Part model, mm, in its own coordinate system. Face numbers are marked on the shaded views. A direction names the side the tool comes from. Round coordinates to 2 decimals unless told otherwise and drop trailing zeros. Write each loop counter-clockwise with the first axis right and the second up, starting at its lowest first coordinate (ties: lowest second). Pieces come first, ordered by that corner, then holes.
```python
from build123d import *

# Parameters (mm, degrees)
BOSS_EXTRUDE1_DEPTH    = 8
SPLIT1_SURFACE_1_BACK  = 343.199
SPLIT1_SURFACE_1_DEPTH = 686.398
SPLIT1_SURFACE_2_BACK  = 343.199
SPLIT1_SURFACE_2_DEPTH = 686.398
SKETCH5_R              = 2.5
CUT_EXTRUDE6_DEPTH     = 5.2
SKETCH4_R              = 2.5
CUT_EXTRUDE7_DEPTH     = 10
SKETCH6_R              = 1.5
CUT_EXTRUDE8_DEPTH     = 342.206659287
SKETCH7_W              = 49
SKETCH7_H              = 49
SKETCH7_W_2            = 18
SKETCH7_H_2            = 18
BOSS_EXTRUDE2_DEPTH    = 15
SKETCH8_W              = 49
SKETCH8_H              = 49
SKETCH8_R              = 1.5
BOSS_EXTRUDE3_DEPTH    = 10
SKETCH9_W              = 49
SKETCH9_H              = 49
CUT_EXTRUDE9_DEPTH     = 8
SKETCH10_W             = 49
SKETCH10_H             = 49
SKETCH10_W_2           = 18
SKETCH10_H_2           = 18
BOSS_EXTRUDE4_DEPTH    = 8
SKETCH12_R             = 2.5
CUT_EXTRUDE10_DEPTH    = 343.027753759


with BuildPart() as part:
    # Sketch1 → Boss-Extrude1 (new body)
    with BuildSketch(Plane.XY):
        with BuildLine():
            Line((70, 309.985818768), (85.299227191, 309.985818768))
            ThreePointArc((85.299227191, 309.985818768), (88.489017574, 308.836174247), (90.211957942, 305.915913694))
            Line((90.211957942, 305.915913694), (96.672728921, 271.790334282))
            ThreePointArc((96.672728921, 271.790334282), (97.06575438, 270.906904614), (97.621470019, 270.115641625))
            Line((97.621470019, 270.115641625), (139.950460317, 220.786053348))
            ThreePointArc((139.950460317, 220.786053348), (141.739336996, 217.746026552), (142.361429131, 214.274017901))
            Line((142.361429131, 214.274017901), (142.361429131, 30.859943174))
            ThreePointArc((142.361429131, 30.859943174), (140.896963037, 27.324409268), (137.361429131, 25.859943174))
            Line((137.361429131, 25.859943174), (114.717190871, 25.782318449))
            ThreePointArc((114.717190871, 25.782318449), (112.681998989, 25.341726514), (111.002773989, 24.110332733))
            Line((111.002773989, 24.110332733), (89.38285929, 0))
            Line((89.38285929, 0), (50.5, 0))
            Line((50.5, 0), (28.997226011, 24.110332733))
            ThreePointArc((28.997226011, 24.110332733), (27.318001011, 25.341726514), (25.282809129, 25.782318449))
            Line((25.282809129, 25.782318449), (2.638570869, 25.859943174))
            ThreePointArc((2.638570869, 25.859943174), (-0.896963037, 27.324409268), (-2.361429131, 30.859943174))
            Line((-2.361429131, 30.859943174), (-2.361429131, 214.274017901))
            ThreePointArc((-2.361429131, 214.274017901), (-1.739336996, 217.746026552), (0.049539683, 220.786053348))
            Line((0.049539683, 220.786053348), (42.261389271, 270.115641625))
            ThreePointArc((42.261389271, 270.115641625), (42.81710491, 270.906904614), (43.210130369, 271.790334282))
            Line((43.210130369, 271.790334282), (49.724618218, 305.923183314))
            ThreePointArc((49.724618218, 305.923183314), (51.449026762, 308.838533573), (54.635967087, 309.985818768))
            Line((54.635967087, 309.985818768), (70, 309.985818768))
        make_face()
        with BuildLine():
            Line((15.218798766, 54.807228462), (17.702103505, 54.807228462))
            ThreePointArc((17.702103505, 54.807228462), (21.420312934, 56.347361236), (22.960445707, 60.065570665))
            Line((22.960445707, 60.065570665), (22.960445707, 189.807228462))
            ThreePointArc((22.960445707, 189.807228462), (21.495979613, 193.342762368), (17.960445707, 194.807228462))
            Line((17.960445707, 194.807228462), (14.960456564, 194.807228462))
            ThreePointArc((14.960456564, 194.807228462), (11.424922658, 193.342762368), (9.960456564, 189.807228462))
            Line((9.960456564, 189.807228462), (9.960456564, 60.065570665))
            ThreePointArc((9.960456564, 60.065570665), (11.500589337, 56.347361236), (15.218798766, 54.807228462))
        make_face(mode=Mode.SUBTRACT)
        with BuildLine():
            Line((125.039543436, 54.807228462), (122.039554293, 54.807228462))
            ThreePointArc((122.039554293, 54.807228462), (118.504020387, 56.271694556), (117.039554293, 59.807228462))
            Line((117.039554293, 59.807228462), (117.039554293, 189.807228462))
            ThreePointArc((117.039554293, 189.807228462), (118.504020387, 193.342762368), (122.039554293, 194.807228462))
            Line((122.039554293, 194.807228462), (125.039543436, 194.807228462))
            ThreePointArc((125.039543436, 194.807228462), (128.575077342, 193.342762368), (130.039543436, 189.807228462))
            Line((130.039543436, 189.807228462), (130.039543436, 59.807228462))
            ThreePointArc((130.039543436, 59.807228462), (128.575077342, 56.271694556), (125.039543436, 54.807228462))
        make_face(mode=Mode.SUBTRACT)
    extrude(amount=BOSS_EXTRUDE1_DEPTH)


with BuildPart() as body_2:
    # Split1: the piece behind the surface
    add(part.part)
    # Split1 surface: a surface, the sketch's curves swept straight by 686.398 mm
    with BuildLine(Plane(origin=(0, 0, 0), x_dir=(-1, 0, 0), z_dir=(0, 0, -1)).offset(-SPLIT1_SURFACE_1_BACK), mode=Mode.PRIVATE) as split1_surface_1_path:
        Line((-142.361429131, 144.05225917), (2.361429131, 144.05225917))
    split1_surface_1 = Shell.extrude(split1_surface_1_path.wire(), (0 * SPLIT1_SURFACE_1_DEPTH, 0 * SPLIT1_SURFACE_1_DEPTH, -1 * SPLIT1_SURFACE_1_DEPTH))
    split(bisect_by=split1_surface_1, keep=Keep.BOTTOM)

    # Sketch5 → Cut-Extrude6 (cut)
    with BuildSketch(Plane(origin=(0, 144.05225917, -115.359943174), x_dir=(1, 0, 0), z_dir=(0, -1, 0))):
        with Locations(Location((70, 119.359943174, 0), (0, 0, 270))):
            Circle(SKETCH5_R)
        with Locations(Location((40, 119.359943174, 0), (0, 0, 270))):
            Circle(SKETCH5_R)
        with Locations(Location((2.638570869, 119.359943174, 0), (0, 0, 270))):
            Circle(SKETCH5_R)
    extrude(amount=CUT_EXTRUDE6_DEPTH, mode=Mode.SUBTRACT)


with BuildPart() as part_1:
    add(part.part)

    # Split1: split by a surface, the side it looks to stays
    # Split1 surface: a surface, the sketch's curves swept straight by 686.398 mm
    with BuildLine(Plane(origin=(0, 0, 0), x_dir=(-1, 0, 0), z_dir=(0, 0, -1)).offset(-SPLIT1_SURFACE_2_BACK), mode=Mode.PRIVATE) as split1_surface_2_path:
        Line((-142.361429131, 144.05225917), (2.361429131, 144.05225917))
    split1_surface_2 = Shell.extrude(split1_surface_2_path.wire(), (0 * SPLIT1_SURFACE_2_DEPTH, 0 * SPLIT1_SURFACE_2_DEPTH, -1 * SPLIT1_SURFACE_2_DEPTH))
    split(bisect_by=split1_surface_2, keep=Keep.TOP)

    # Sketch4 → Cut-Extrude7 (cut)
    with BuildSketch(Plane(origin=(0, 144.05225917, 0), x_dir=(-1, 0, 0), z_dir=(0, -1, 0))):
        with Locations(Location((-70, -4, 0), (0, 0, 270))):
            Circle(SKETCH4_R)
        with Locations(Location((-40, -4, 0), (0, 0, 270))):
            Circle(SKETCH4_R)
        with Locations(Location((-100, -4, 0), (0, 0, 270))):
            Circle(SKETCH4_R)
        with Locations(Location((-137.361429131, -4, 0), (0, 0, 90))):
            Circle(SKETCH4_R)
        with Locations(Location((-3.799513716, -4, 0), (0, 0, 270))):
            Circle(SKETCH4_R)
    extrude(amount=-CUT_EXTRUDE7_DEPTH, mode=Mode.SUBTRACT)

    # Sketch6 → Cut-Extrude8 (cut, through all)
    with BuildSketch(Plane.XY.offset(8)):
        with Locations((50.000130369, 267.980334282)):
            Circle(SKETCH6_R)
        with Locations((90.000130369, 267.980334282)):
            Circle(SKETCH6_R)
        with Locations((90.000130369, 227.980334282)):
            Circle(SKETCH6_R)
        with Locations((50.000130369, 227.980334282)):
            Circle(SKETCH6_R)
    extrude(amount=-CUT_EXTRUDE8_DEPTH, mode=Mode.SUBTRACT)

    # Sketch7 → Boss-Extrude2 (add)
    with BuildSketch(Plane(origin=(0, 0, 0), x_dir=(-1, 0, 0), z_dir=(0, 0, -1))):
        with Locations((-70.000130369, 247.980334282)):
            Rectangle(SKETCH7_W, SKETCH7_H)
        with Locations((-56.000130369, 261.980334282)):
            Rectangle(SKETCH7_W_2, SKETCH7_H_2, mode=Mode.SUBTRACT)
        with Locations((-84.000130369, 261.980334282)):
            Rectangle(SKETCH7_W_2, SKETCH7_H_2, mode=Mode.SUBTRACT)
        with Locations((-84.000130369, 233.980334282)):
            Rectangle(SKETCH7_W_2, SKETCH7_H_2, mode=Mode.SUBTRACT)
        with Locations((-56.000130369, 233.980334282)):
            Rectangle(SKETCH7_W_2, SKETCH7_H_2, mode=Mode.SUBTRACT)
    extrude(amount=BOSS_EXTRUDE2_DEPTH)

    # Sketch8 → Boss-Extrude3 (add)
    with BuildSketch(Plane(origin=(0, 0, -15), x_dir=(-1, 0, 0), z_dir=(0, 0, -1))):
        with Locations((-70.000130369, 247.980334282)):
            Rectangle(SKETCH8_W, SKETCH8_H)
        with Locations(Location((-50.000130369, 267.980334282, 0), (0, 0, 180))):
            Circle(SKETCH8_R, mode=Mode.SUBTRACT)
        with Locations(Location((-90.000130369, 267.980334282, 0), (0, 0, 180))):
            Circle(SKETCH8_R, mode=Mode.SUBTRACT)
        with Locations(Location((-50.000130369, 227.980334282, 0), (0, 0, 180))):
            Circle(SKETCH8_R, mode=Mode.SUBTRACT)
        with Locations(Location((-90.000130369, 227.980334282, 0), (0, 0, 180))):
            Circle(SKETCH8_R, mode=Mode.SUBTRACT)
    extrude(amount=BOSS_EXTRUDE3_DEPTH)

    # Sketch9 → Cut-Extrude9 (cut)
    with BuildSketch(Plane.XY.offset(8)):
        with Locations((70.000130369, 247.980334282)):
            Rectangle(SKETCH9_W, SKETCH9_H)
    extrude(amount=-CUT_EXTRUDE9_DEPTH, mode=Mode.SUBTRACT)


with BuildPart() as cut_extrude9_piece_1:
    # of the separate pieces the step leaves, piece 1, a body of its own (cut_extrude9_pieces)
    add(part_1.part.solids().sort_by_distance((49.724618218, 305.923183314, 0))[0])



with BuildPart() as cut_extrude9_piece_2:
    # of the separate pieces the step leaves, piece 2, a body of its own (cut_extrude9_pieces)
    add(part_1.part.solids().sort_by_distance((45.500130369, 223.480334282, -25))[0])


with BuildPart() as cut_extrude9_piece_1_1:
    add(cut_extrude9_piece_1.part)

    add(cut_extrude9_piece_2.part)  # Boss-Extrude4 merges Cut-Extrude9 piece 2
    # Sketch10 → Boss-Extrude4 (add)
    with BuildSketch(Plane.XY):
        with Locations((70.000130369, 247.980334282)):
            Rectangle(SKETCH10_W, SKETCH10_H)
        with Locations((84.000130369, 261.980334282)):
            Rectangle(SKETCH10_W_2, SKETCH10_H_2, mode=Mode.SUBTRACT)
        with Locations((56.000130369, 261.980334282)):
            Rectangle(SKETCH10_W_2, SKETCH10_H_2, mode=Mode.SUBTRACT)
        with Locations((56.000130369, 233.980334282)):
            Rectangle(SKETCH10_W_2, SKETCH10_H_2, mode=Mode.SUBTRACT)
        with Locations((84.000130369, 233.980334282)):
            Rectangle(SKETCH10_W_2, SKETCH10_H_2, mode=Mode.SUBTRACT)
    extrude(amount=BOSS_EXTRUDE4_DEPTH)

    # Sketch12 → Cut-Extrude10 (cut, through all)
    with BuildSketch(Plane(origin=(0, 0, 0), x_dir=(-1, 0, 0), z_dir=(0, 0, -1))):
        with Locations((-102.960445707, 197.503395095)):
            Circle(SKETCH12_R)
        with Locations((-35.960445707, 197.503395095)):
            Circle(SKETCH12_R)
        with Locations((-35.960445707, 157.503395095)):
            Circle(SKETCH12_R)
        with Locations((-102.960445707, 157.503395095)):
            Circle(SKETCH12_R)
    extrude(amount=-CUT_EXTRUDE10_DEPTH, mode=Mode.SUBTRACT)


solid = cut_extrude9_piece_1_1.part
```
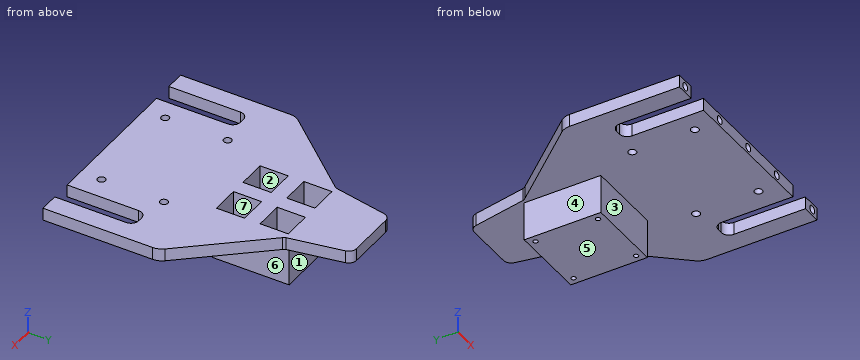
Q1. Cut at A-A on y = 164.5. Write the cut outline in (x, z).
Values follow:
outline: (-2.36, 0) - (9.96, 0) - (9.96, 8) - (-2.36, 8) - close; (22.96, 0) - (117.04, 0) - (117.04, 8) - (22.96, 8) - close; (130.04, 0) - (142.36, 0) - (142.36, 8) - (130.04, 8) - close
Q2. Drop flat-ended pins along their axis: pin 1 (14.5 mm diameter, centred on x = 81, z = -7, fed in from -Y); pin 2 (4 mm diameter, centred on x = 102.96, y = 157.5, fed in from -Z); pin 3 (10 mm diameter, centred on y = 241.5, z = -10, fed in from -X); pin 4 (2 mm diameter, centred on x = 65.5, z = -16, fed in from +Y). Give the stop position or say it passes through.
Values follow:
pin 1: stops at y = 144.05
pin 2: passes through
pin 3: stops at x = 45.5
pin 4: stops at y = 272.48
Q3. Wall check: L1, parallel to Y at x = 50, z = -6; L2, parallel to Y at x = 52, z = 2; L3, parallel to Z at x = 39, y = 185. Give the ranges that are in metal, low to high.
Values follow:
L1: y = 223.48 to 224.98, 242.98 to 252.98, 270.98 to 272.48
L2: y = 144.05 to 224.98, 242.98 to 252.98, 270.98 to 309.23
L3: z = 0 to 8
Q4. Which spindle directions (+Z, -Z, +X, -X, +Y, -Y) get a long thin tool onto all of the face, cutting with end or side? Do the marked faces 1, 2 and 3. Say none if no direction does.
Values follow:
face 1: -Z, +X, -X, +Y
face 2: +Z
face 3: -Z, +X, -X, -Y
Q5. Cut at B-B on z = -2. Write the cut outline in (x, y), plus the area to 4 significant figures.
Values follow:
outline: (45.5, 223.48) - (94.5, 223.48) - (94.5, 272.48) - (45.5, 272.48) - close; hole (47, 224.98) - (65, 224.98) - (65, 242.98) - (47, 242.98) - close; hole (47, 252.98) - (65, 252.98) - (65, 270.98) - (47, 270.98) - close; hole (75, 224.98) - (93, 224.98) - (93, 242.98) - (75, 242.98) - close; hole (75, 252.98) - (93, 252.98) - (93, 270.98) - (75, 270.98) - close
area: 1,105 mm2
Q6. Mould opens along X. For the marked faces 4, 5, 6 and 7 say: +X half, -X half, draft (parallel to the pull), parting line (faces both ways), or undercut.
Values follow:
face 4: -X half
face 5: draft
face 6: +X half
face 7: undercut
Q7. Cut at C-C on x = 35.5. Write the cut outline in (y, z), plus the area to 3 significant figures.
Values follow:
outline: (144.05, 0) - (155.05, 0) - (155.05, 8) - (144.05, 8) - close; (159.96, 0) - (195.05, 0) - (195.05, 8) - (159.96, 8) - close; (199.96, 0) - (262.21, 0) - (262.21, 8) - (199.96, 8) - close
area: 867 mm2
Q8. Cut at D-D on x = 70. Write the cut outline in (y, z).
Values follow:
outline: (144.05, 0) - (223.48, 0) - (223.48, -25) - (272.48, -25) - (272.48, 0) - (309.99, 0) - (309.99, 8) - (144.05, 8) - (144.05, 6.5) - (154.05, 6.5) - (154.05, 1.5) - (144.05, 1.5) - close
